For this review, take the finished solid that the model builds, in its own axes (mm). A direction names the side the tool comes from. Give positions to 0.01 mm unless a question says otherwise; leave off trailing zeros. Loops run counter-clockwise (first coordinate to the right, second up) from the corner with the lowest first, then second, coordinate; pieces in that order, holes last. Notation, with made-up numbers: M 57.5,28 L 97.5,28 A18 cw 97.5,50 Z; hole C 66,86 d1. An arc over 180 degrees is marked long. Use CSV: the item, a comma, the result in double quotes. Start each with the question number.
1. Take a section at B-B, the plane x = 1.5. Write out the cut boundary in (y, z).
2. The part is to be moulded in two halves that separate along X. For faces 1 (the face through (2.03, 14.1, 0.86)), 2 (the face through (7, 6, 11)), 3 (the face through (11.5, 3, 8.6)), say which applies: pulls with the +X half, pulls with the -X half, needs draft (parallel to the pull), parting line crosses it, or undercut.
3. Tool access review of faces 4 (the face through (3, 12.1, 7.5)), 5 (the face through (9.3, 2, 7.5)), 6 (the face through (6, 6, 2)): name each direction out of +Z, -Z, +X, -X, +Y, -Y from which nothing blocks a thin tool from reaching the whole face with its end or side.
4. Take a section at A-A, the plane y = 2.5. Write out the cut boundary in (x, z).
5. Take a section at D-D, the plane z = 8. Write out the cut boundary in (x, y), and give its area (3 significant figures).
6. Insertion check: P1, Ø6.5, axis at x = 11.5, z = 6.5, coming from the +Y side; P2, Ø1.8, axis at y = 9.5, z = 6, coming from the +X side; P3, Ø5.5, axis at y = 9.5, z = 7.5, coming from the +X side; P4, Ø1.9, axis at x = 6, y = 8, coming from the +Z side. Each pin has a flat end and moves straight along its axis. Give the tip position at first contact, or say it passes through.
7. Take a section at C-C, the plane y = 9.5. Write out the cut boundary in (x, z), and give its area (3 significant figures).
8. To check wall thickness, follow line 1 (Z direction, x = 1.65, y = 9.5); line 2 (Z direction, x = 5, y = 4.5); line 3 (Y direction, x = 3.5, z = 7.25). State the ranges of each line that lie inside material, in increasing order. Write a range as [from, to].
from build123d import *

# Parameters (mm, degrees)
BOSS_EXTRUDE1_DEPTH = 12
SKETCH2_R           = 1.5
CUT_EXTRUDE1_DEPTH  = 23.649503306
CUT_EXTRUDE2_DEPTH  = 2
SKETCH4_R           = 1.5
CUT_EXTRUDE3_DEPTH  = 26
CUT_EXTRUDE4_DEPTH  = 2
BOSS_EXTRUDE2_DEPTH = 2
BOSS_EXTRUDE3_DEPTH = 2
FILLET1_R           = 3


with BuildPart() as part:
    # Sketch1 → Boss-Extrude1 (new body)
    with BuildSketch(Plane.XY):
        Polygon((0, 0), (0, 15), (4, 15), (4, 4), (16, 4), (16, 0), align=None)
    extrude(amount=BOSS_EXTRUDE1_DEPTH)

    # Sketch2 → Cut-Extrude1 (cut, through all)
    with BuildSketch(Plane(origin=(4, 0, 0), x_dir=(0, 0, -1), z_dir=(1, 0, 0))):
        with Locations(Location((-6, 9.5, 0), (0, 0, 90))):
            Circle(SKETCH2_R)
    extrude(amount=-CUT_EXTRUDE1_DEPTH, mode=Mode.SUBTRACT)

    # Sketch3 → Cut-Extrude2 (cut)
    with BuildSketch(Plane(origin=(4, 0, 0), x_dir=(0, 0, -1), z_dir=(1, 0, 0))):
        Polygon((-6, 12.964101615), (-9, 11.232050808), (-9, 7.767949192), (-6, 6.035898385), (-3, 7.767949192), (-3, 11.232050808), align=None)
    extrude(amount=-CUT_EXTRUDE2_DEPTH, mode=Mode.SUBTRACT)

    # Sketch4 → Cut-Extrude3 (cut, through all)
    with BuildSketch(Plane.XZ):
        with Locations((10, 6)):
            Circle(SKETCH4_R)
    extrude(amount=-CUT_EXTRUDE3_DEPTH, mode=Mode.SUBTRACT)

    # Sketch5 → Cut-Extrude4 (cut)
    with BuildSketch(Plane(origin=(0, 4, 0), x_dir=(1, 0, 0), z_dir=(0, 1, 0))):
        Polygon((10, -9.464101615), (13, -7.732050808), (13, -4.267949192), (10, -2.535898385), (7, -4.267949192), (7, -7.732050808), align=None)
    extrude(amount=-CUT_EXTRUDE4_DEPTH, mode=Mode.SUBTRACT)

    # Sketch6 → Boss-Extrude2 (add)
    with BuildSketch(Plane(origin=(0, 0, 0), x_dir=(-1, 0, 0), z_dir=(0, 0, -1))):
        Polygon((-4, 4), (-4, 9), (-9, 4), align=None)
    extrude(amount=-BOSS_EXTRUDE2_DEPTH)

    # Sketch7 → Boss-Extrude3 (add)
    with BuildSketch(Plane.XY.offset(12)):
        Polygon((4, 9), (4, 4), (9, 4), align=None)
    extrude(amount=-BOSS_EXTRUDE3_DEPTH)

    # Fillet1
    fillet1_edges = [part.edges().sort_by_distance(p)[0] for p in [
        (2, 15, 12),
        (2, 15, 0),
        (16, 2, 12),
        (9, 4, 1),
        (4, 9, 1),
        (16, 2, 0),
        (9, 4, 11),
        (4, 9, 11),
    ]]
    fillet(fillet1_edges, radius=FILLET1_R)


solid = part.part
Result set:
1,outline,"M 0,0 L 12,0 A3 ccw 15,3 L 15,9 A3 ccw 12,12 L 0,12 Z; hole C 9.5,6 d3"
2,face 1,"needs draft"
2,face 2,"pulls with the +X half"
2,face 3,"undercut"
3,face 4,"+X"
3,face 5,"+Y"
3,face 6,"+X, +Y"
4,outline,"M 0,0 L 13,0 A3 ccw 16,3 L 16,9 A3 ccw 13,12 L 0,12 Z; hole M 7,4.27 L 10,2.54 L 13,4.27 L 13,7.73 L 10,9.46 L 7,7.73 Z"
5,outline,"M 0,0 L 16,0 L 16,4 L 12.54,4 L 12.54,2 L 7.46,2 L 7.46,4 L 4,4 L 4,7.19 L 2,7.19 L 2,11.81 L 4,11.81 L 4,15 L 0,15 Z"
5,area,"88.6 mm2"
6,P1,"y = 4"
6,P2,"through"
6,P3,"x = 4.67"
6,P4,"z = 12"
7,outline,"M 0,0 L 4.09,0 L 4.09,2 L 4,2 L 4,3 L 2,3 L 2,4.5 L 0,4.5 Z; M 0,7.5 L 2,7.5 L 2,9 L 4,9 L 4,10 L 4.09,10 L 4.09,12 L 0,12 Z"
7,area,"30.4 mm2"
8,line 1,"[0, 4.5], [7.5, 12]"
8,line 2,"[0, 2], [10, 12]"
8,line 3,"[0, 6.76], [12.24, 15]"
